```python
from build123d import *


with BuildPart() as part:
    # Skica1 → Rotovat1 (revolve)
    with BuildSketch(Plane(origin=(0, 0, 0), x_dir=(1, 0, 0), z_dir=(0, 1, 0))):
        with BuildLine():
            Line((9.5, 0), (9.5, 25))
            Line((9.5, 25), (0, 25))
            Line((0, 25), (0, -1.929477619))
            ThreePointArc((0, -1.929477619), (3.894000592, -1.650357757), (7.70838162, -0.818705261))
            Line((7.70838162, -0.818705261), (7.70838162, -0.488101593))
            Line((7.70838162, -0.488101593), (7.939207246, -0.488101593))
            Line((7.939207246, -0.488101593), (7.939207246, -0.761243378))
            Line((7.939207246, -0.761243378), (11, -0.082108279))
            Line((11, -0.082108279), (11, 0))
            Line((11, 0), (9.5, 0))
        make_face()
    revolve(axis=Axis((0, 0, 3.381080674), (0, 0, -1)))


solid = part.part
```
The listing builds one solid part. Answer for the finished solid, in the listing's coordinates (mm). Give positions to 0.01 mm unless a question says otherwise; leave off trailing zeros. Order: outer loops, then holes, each group sorted by start corner. A loop starts at its lowest first (then second) coordinate and runs counter-clockwise, first axis right, second up. Notation, with made-up numbers: (58, -13.75) - (113, -13.75) arc R24 cw to (113, 19.25) - close; hole circle Ø3 at (6, -20.75). An arc over 180 degrees is marked (long way). Answer in a Markdown table with one row per item. Add a question column.
Q1. Find the intervals of material crossed by line 1 along Z through (x, y) = (5.5, -3); line 2 along Z through (x, y) = (-8, -5); line 3 along Y through (x, z) = (0.75, -17.5), in increasing order. Write a range as [from, to].
Q2. The part is cut by section C-C (z = -12.5). Determine the outline of the cut face in (x, y), then the cut area to 3 significant figures.
Q3. The part is cut by section A-A (y = 0). Determine the outline of the cut face in (x, z), then the cut area to 3 significant figures.
Q4. Given P1, Ø1, axis at y = -4, z = -3.5, coming from the +X side; P2, Ø3, axis at x = -6.5, z = -11, coming from the +Y side; P3, Ø8, axis at y = 8.5, z = -22, coming from the -X side, each flat-ended and moving along its own axis, determine where each tip first touches the part or whether it passes through.
Q5. For a pull along Y with two mould halves and no side action, classify faces 1 (the flat face through (-10, 0, 0)), 2 (the cylindrical face through (4.38, 8.43, -12.68)), 3 (the cylindrical face through (-1.671, 7.525, 0.651)) as released by +Y, released by -Y, zero draft, split by the parting line, or undercut.
Determined:
| question | item | result |
|---|---|---|
| 1 | line 1 | z = [-25, 1.2] |
| 1 | line 2 | z = [-25, 0.43] |
| 1 | line 3 | y = [-9.47, 9.47] |
| 2 | outline | circle Ø19 at (0, 0) |
| 2 | area | 284 mm² |
| 3 | outline | (-11, 0) - (-9.5, 0) - (-9.5, -25) - (9.5, -25) - (9.5, 0) - (11, 0) - (11, 0.08) - (7.94, 0.76) - (7.94, 0.49) - (7.71, 0.49) - (7.71, 0.82) arc R27.3 ccw to (-7.71, 0.82) - (-7.71, 0.49) - (-7.94, 0.49) - (-7.94, 0.76) - (-11, 0.08) - close |
| 3 | area | 502 mm² |
| 4 | P1 | stops at x = 8.83 |
| 4 | P2 | stops at y = 8.08 |
| 4 | P3 | stops at x = -8.37 |
| 5 | face 1 | zero draft |
| 5 | face 2 | split by the parting line |
| 5 | face 3 | undercut |
